Source: CAD feature listing. Evaluate the final solid. Frame: model axes, mm. Give positions to 0.01 mm unless a question says otherwise; leave off trailing zeros. Loops run counter-clockwise (first coordinate to the right, second up) from the corner with the lowest first, then second, coordinate; pieces in that order, holes last. Notation, with made-up numbers: (-32.75, 13.25) - (11.25, 13.25) arc R30 ccw to (11.25, 35.25) - close; hole circle Ø11 at (23, 87.5). An arc over 180 degrees is marked (long way). Write each question's results on one line, items separated by ' | '. Start each with the question number.
(1) Pull-direction query (Y, two-part tool) for faces 1 (the cylindrical face through (-86.023, 14.589, 0.986)), 2 (the flat face through (-11, 0, 2)); classes: pulls with the +Y half, pulls with the -Y half, needs draft (parallel to the pull), parting line crosses it, or undercut.
(2) Cut plane B-B on y = 14.5. Return the cut outline in (x, z) (3 decimals), then the cut area to 3 significant figures.
(3) Cut plane C-C on x = 64. Return the cut outline in (y, z) (3 decimals), then the cut area to 3 significant figures.
(4) Material intervals for line 1 along Y through (x, z) = (64, 0.6) (3 decimals); line 2 along Y through (x, z) = (52.5, 0.55) (3 decimals); line 3 along Y through (x, z) = (-52.5, 1.3) (3 decimals), sorted ascending. Write a range as [from, to].
(5) Cut plane A-A on x = -84. Return the cut outline in (y, z) (3 decimals).
(6) Contact query for flat-ended pins moving along their axis: pin 1 (5 mm diameter, centred on x = -52.5, y = 14.5, fed in from +Z); pin 2 (2.5 mm diameter, centred on x = 52.5, y = -14.5, fed in from -Z); pin 3 (0.6 mm diameter, centred on y = -1, z = 1, fed in from -X). Output: stop coordinate, or through.
(7) Cut plane D-D on z = 0.35. Give the number of separate pieces and of enclosed holes in the cut face, then the cut area to 3 significant figures.
from build123d import *

# Parameters (mm, degrees)
SKETCH_1_W          = 32
SKETCH_1_H          = 39
SKETCH_1_R          = 2.025
SKETCH_1_W_2        = 115
SKETCH_1_R_2        = 1.525
SKETCH_1_W_3        = 12
EXTRUDE_1_DEPTH     = 2
SKETCH_2_W          = 19
SKETCH_2_H          = 15
SKETCH_2_W_2        = 26
CUT_EXTRUDE_1_DEPTH = 10
FILLET_1_R          = 2


with BuildPart() as part:
    # 草图1 → 凸台-拉伸1 (new body)
    with BuildSketch(Plane.XY):
        with Locations((-73.5, 0)):
            Rectangle(SKETCH_1_W, SKETCH_1_H)
        with Locations((-84, -14.5)):
            Circle(SKETCH_1_R, mode=Mode.SUBTRACT)
        with Locations((-84, 14.5)):
            Circle(SKETCH_1_R, mode=Mode.SUBTRACT)
        Rectangle(SKETCH_1_W_2, SKETCH_1_H)
        with Locations((52.5, 14.5)):
            Circle(SKETCH_1_R_2, mode=Mode.SUBTRACT)
        with Locations((52.5, -14.5)):
            Circle(SKETCH_1_R_2, mode=Mode.SUBTRACT)
        with Locations((-52.5, -14.5)):
            Circle(SKETCH_1_R_2, mode=Mode.SUBTRACT)
        with Locations((-52.5, 14.5)):
            Circle(SKETCH_1_R_2, mode=Mode.SUBTRACT)
        with Locations((63.5, 0)):
            Rectangle(SKETCH_1_W_3, SKETCH_1_H)
        with Locations((64, -14.5)):
            Circle(SKETCH_1_R, mode=Mode.SUBTRACT)
        with Locations((64, 14.5)):
            Circle(SKETCH_1_R, mode=Mode.SUBTRACT)
    extrude(amount=EXTRUDE_1_DEPTH)

    # 草图2 → 切除-拉伸1 (cut)
    with BuildSketch(Plane.XY.offset(2)):
        with Locations((-80, 0)):
            Rectangle(SKETCH_2_W, SKETCH_2_H)
        with Locations((-57.5, 0)):
            Rectangle(SKETCH_2_W_2, SKETCH_2_H)
    extrude(amount=-CUT_EXTRUDE_1_DEPTH, mode=Mode.SUBTRACT)

    # 圆角1
    fillet_1_edges = [part.edges().sort_by_distance(p)[0] for p in [
        (-89.5, 19.5, 1),
        (69.5, 19.5, 1),
        (69.5, -19.5, 1),
        (-89.5, -19.5, 1),
        (-44.5, -7.5, 1),
        (-89.5, -7.5, 1),
        (-89.5, 7.5, 1),
        (-44.5, 7.5, 1),
    ]]
    fillet(fillet_1_edges, radius=FILLET_1_R)


solid = part.part
Ans:
1) face 1: undercut | face 2: needs draft
2) outline: (-89.5, 0) - (-86.025, 0) - (-86.025, 2) - (-89.5, 2) - close; (-81.975, 0) - (-54.025, 0) - (-54.025, 2) - (-81.975, 2) - close; (-50.975, 0) - (50.975, 0) - (50.975, 2) - (-50.975, 2) - close; (54.025, 0) - (61.975, 0) - (61.975, 2) - (54.025, 2) - close; (66.025, 0) - (69.5, 0) - (69.5, 2) - (66.025, 2) - close | area: 290 mm^2
3) outline: (-19.5, 0) - (-16.525, 0) - (-16.525, 2) - (-19.5, 2) - close; (-12.475, 0) - (12.475, 0) - (12.475, 2) - (-12.475, 2) - close; (16.525, 0) - (19.5, 0) - (19.5, 2) - (16.525, 2) - close | area: 61.8 mm^2
4) line 1: [-19.5, -16.525], [-12.475, 12.475], [16.525, 19.5] | line 2: [-19.5, -16.025], [-12.975, 12.975], [16.025, 19.5] | line 3: [-19.5, -16.025], [-12.975, -7.5], [7.5, 12.975], [16.025, 19.5]
5) outline: (-19.5, 0) - (-16.525, 0) - (-16.525, 2) - (-19.5, 2) - close; (-12.475, 0) - (-7.5, 0) - (-7.5, 2) - (-12.475, 2) - close; (7.5, 0) - (12.475, 0) - (12.475, 2) - (7.5, 2) - close; (16.525, 0) - (19.5, 0) - (19.5, 2) - (16.525, 2) - close
6) pin 1: z = 2 | pin 2: through | pin 3: x = -44.5
7) separate pieces: 1 | enclosed holes: 8 | area: 5,440 mm^2
